The listing builds one solid part. Answer for the finished solid, in the listing's coordinates (mm). Face numbers are marked on the shaded views. A direction names the side the tool comes from. Coordinates: 2 decimals unless noted, no trailing zeros. Write each loop counter-clockwise with the first axis right and the second up, starting at its lowest first coordinate (ties: lowest second). Pieces come first, ordered by that corner, then holes.
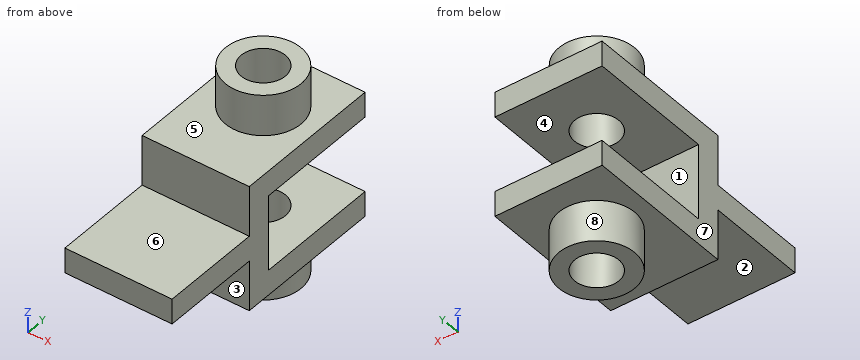
from build123d import *

# Parameters (mm, degrees)
SALIENTE_EXTRUIR1_DEPTH = 17
CROQUIS10_R             = 7
CORTAR_EXTRUIR2_DEPTH   = 92.043945433
SALIENTE_EXTRUIR5_START = 13
CROQUIS11_R             = 12
CROQUIS11_R_2           = 7
SALIENTE_EXTRUIR5_DEPTH = 13
CROQUIS12_R             = 12
CROQUIS12_R_2           = 7
SALIENTE_EXTRUIR6_DEPTH = 13


with BuildPart() as part:
    # Croquis1 → Saliente-Extruir1 (new, symmetric)
    with BuildSketch(Plane(origin=(0, 0, 0), x_dir=(0, 0, -1), z_dir=(1, 0, 0))):
        Polygon((0, 0), (0, 32), (-16, 32), (-16, 80), (-8, 80), (-8, 40), (16, 40), (16, 80), (24, 80), (24, 32), (8, 32), (8, 0), align=None)
    extrude(amount=SALIENTE_EXTRUIR1_DEPTH, both=True)

    # Croquis10 → Cortar-Extruir2 (cut, through all)
    with BuildSketch(Plane.XY.offset(16)):
        with Locations((0, 60)):
            Circle(CROQUIS10_R)
    extrude(amount=-CORTAR_EXTRUIR2_DEPTH, mode=Mode.SUBTRACT)

    # Croquis11 → Saliente-Extruir5 (add)
    with BuildSketch(Plane.XY.offset(16).offset(SALIENTE_EXTRUIR5_START)):
        with Locations(Location((0, 60, 0), (0, 0, 180))):
            Circle(CROQUIS11_R)
        with Locations((0, 60)):
            Circle(CROQUIS11_R_2, mode=Mode.SUBTRACT)
    extrude(amount=-SALIENTE_EXTRUIR5_DEPTH)

    # Croquis12 → Saliente-Extruir6 (add)
    with BuildSketch(Plane(origin=(0, 0, -24), x_dir=(-1, 0, 0), z_dir=(0, 0, -1))):
        with Locations((0, 60)):
            Circle(CROQUIS12_R)
        with Locations(Location((0, 60, 0), (0, 0, 180))):
            Circle(CROQUIS12_R_2, mode=Mode.SUBTRACT)
    extrude(amount=SALIENTE_EXTRUIR6_DEPTH)


solid = part.part
Q1. Given pin 1 (3 mm diameter, centred on y = 29, z = -18.5, fed in from -X); pin 2 (6 mm diameter, centred on x = 9, y = 36, fed in from +Z); pin 3 (16 mm diameter, centred on x = 7, y = 19.5, fed in from -Z); pin 4 (16 mm diameter, centred on x = -5, y = 23, fed in from +Z), each flat-ended and moving along its own axis, determine where each tip first touches the part or whether it passes through.
Answers below:
pin 1: passes through
pin 2: stops at z = 16
pin 3: stops at z = -8
pin 4: stops at z = 0
Q2. Which of the six approach directions +Z, -Z, +X, -X, +Y, -Y give full straight-line access (tool end or side, diameter ignored) to the marked faces 5, 6, 7 and 8?
Answers below:
face 5: +Z
face 6: +Z, +X, -X, -Y
face 7: +Z, -Z, -X, +Y, -Y
face 8: -Z
Q3. Determine the mould class of the marked faces 1, 2, 3 and 4 for opening direction Z: released by +Z, released by -Z, zero draft, split by the parting line, or undercut.
Answers below:
face 1: undercut
face 2: released by -Z
face 3: zero draft
face 4: undercut
Q4. The part is cut by section C-C, the plane x = 6. Write down the section's boundary in (y, z), then the cut area to 3 significant figures.
Answers below:
outline: (0, -8) - (32, -8) - (32, -24) - (49.61, -24) - (49.61, -37) - (56.39, -37) - (56.39, -16) - (40, -16) - (40, 8) - (56.39, 8) - (56.39, 29) - (49.61, 29) - (49.61, 16) - (32, 16) - (32, 0) - (0, 0) - close; (63.61, -37) - (70.39, -37) - (70.39, -24) - (80, -24) - (80, -16) - (63.61, -16) - close; (63.61, 8) - (80, 8) - (80, 16) - (70.39, 16) - (70.39, 29) - (63.61, 29) - close
area: 1,450 mm2
Q5. The part is cut by section D-D, the plane z = -14.5. Write down the section's boundary in (x, y), then the cut area to 3 significant figures.
Answers below:
outline: (-17, 32) - (17, 32) - (17, 40) - (-17, 40) - close
area: 272 mm2
Q6. The part is cut by section B-B, the plane z = 15. Write down the section's boundary in (x, y).
Answers below:
outline: (-17, 32) - (17, 32) - (17, 80) - (-17, 80) - close; hole circle Ø14 at (0, 60)
Q7. Find the intervals of material crossed by probe 1 along Y at (x, z) = (0, -26); probe 2 along Z at (x, y) = (10, 54); probe 3 along Y at (x, z) = (0, -23.5), in increasing order.
Answers below:
probe 1: y = 48 to 53, 67 to 72
probe 2: z = -37 to -16, 8 to 29
probe 3: y = 32 to 53, 67 to 80
Q8. The part is cut by section A-A, the plane y = 62.5. Write down the section's boundary in (x, z), then the cut area to 3 significant figures.
Answers below:
outline: (-17, -24) - (-11.74, -24) - (-11.74, -37) - (-6.54, -37) - (-6.54, -16) - (-17, -16) - close; (-17, 8) - (-6.54, 8) - (-6.54, 29) - (-11.74, 29) - (-11.74, 16) - (-17, 16) - close; (6.54, -37) - (11.74, -37) - (11.74, -24) - (17, -24) - (17, -16) - (6.54, -16) - close; (6.54, 8) - (17, 8) - (17, 16) - (11.74, 16) - (11.74, 29) - (6.54, 29) - close
area: 605 mm2
